from build123d import *

# Parameters (mm, degrees)
SKETCH_1_R      = 1.5
EXTRUDE_1_DEPTH = 3


with BuildPart() as part:
    # 草图1 → 凸台-拉伸1 (new body)
    with BuildSketch(Plane(origin=(0, 0, 0), x_dir=(0, 0, -1), z_dir=(1, 0, 0))):
        Polygon((0, 0), (240, 0), (240, -20), (158, -20), (158, -152), (139, -152), (139, -20), (101, -20), (101, -152), (82, -152), (82, -20), (0, -20), align=None)
        with Locations((72.5, -14)):
            Circle(SKETCH_1_R, mode=Mode.SUBTRACT)
        with Locations((110.5, -14)):
            Circle(SKETCH_1_R, mode=Mode.SUBTRACT)
        with Locations((129.5, -14)):
            Circle(SKETCH_1_R, mode=Mode.SUBTRACT)
        with Locations((167.5, -14)):
            Circle(SKETCH_1_R, mode=Mode.SUBTRACT)
        with Locations((10, -10)):
            Circle(SKETCH_1_R, mode=Mode.SUBTRACT)
        with Locations((230, -10)):
            Circle(SKETCH_1_R, mode=Mode.SUBTRACT)
        with Locations((37.52, -10)):
            Circle(SKETCH_1_R, mode=Mode.SUBTRACT)
        with Locations((202.48, -10)):
            Circle(SKETCH_1_R, mode=Mode.SUBTRACT)
    extrude(amount=EXTRUDE_1_DEPTH)


solid = part.part
Read the model definition and answer for the solid it produces. Units are mm, in the model's axes. Round coordinates to 2 decimals unless told otherwise and drop trailing zeros. Order: outer loops, then holes, each group sorted by start corner. A loop starts at its lowest first (then second) coordinate and runs counter-clockwise, first axis right, second up.
1) Straight lines are drawn through the part: L1, parallel to Z at x = 2.45, y = -79.5; L2, parallel to Y at x = 1.85, z = -202.48; L3, parallel to Y at x = 0.9, z = -69.5. For each, find the intervals that lie inside material, in ascending order.
2) The part is cut by section B-B on y = -109. Write down the section's boundary in (x, z), plus the area to 3 significant figures.
3) The part is cut by section A-A on x = 2. Give the number of separate pieces and of enclosed holes in the cut face, plus the area to 3 significant figures.
4) The part is cut by section C-C on z = -222.5. Write down the section's boundary in (x, y).
5) Flat-ended cylindrical pins translate along their axes: pin 1 (2.5 mm diameter, centred on y = -10, z = -10, fed in from +X); pin 2 (3.5 mm diameter, centred on y = -14, z = -110.5, fed in from -X); pin 3 (0.9 mm diameter, centred on x = 1.5, y = -79.5, fed in from +Z); pin 4 (1 mm diameter, centred on x = 2.5, y = -102, fed in from -Z). Find the tip coordinate at first contact, or state that the pin passes through.
Resolved:
1. L1: z = -158 to -139, -101 to -82
1. L2: y = -20 to -11.5, -8.5 to 0
1. L3: y = -20 to 0
2. outline: (0, -158) - (3, -158) - (3, -139) - (0, -139) - close; (0, -101) - (3, -101) - (3, -82) - (0, -82) - close
2. area: 114 mm2
3. separate pieces: 1
3. enclosed holes: 8
3. area: 9,760 mm2
4. outline: (0, -20) - (3, -20) - (3, 0) - (0, 0) - close
5. pin 1: passes through
5. pin 2: stops at x = 0
5. pin 3: stops at z = -82
5. pin 4: stops at z = -158
